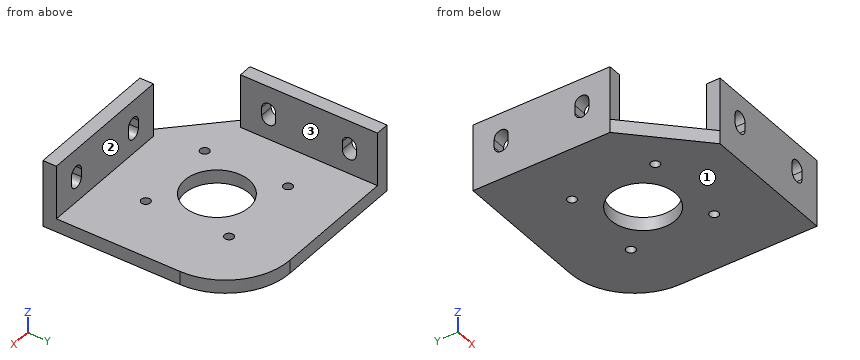
```python
from build123d import *

# Parameters (mm, degrees)
PAD_DEPTH       = 5
SKETCH002_R     = 1.68
SKETCH002_R_2   = 12
POCKET_DEPTH    = 5
FILLET_R        = 24
SKETCH_W        = 5
SKETCH_H        = 51
SKETCH_W_2      = 51
SKETCH_H_2      = 5
PAD001_DEPTH    = 20
POCKET001_DEPTH = 5
POCKET002_DEPTH = 5


with BuildPart() as part:
    # Sketch001 → Pad (new body)
    with BuildSketch(Plane.XY):
        Polygon((75, 0), (75, 75), (0, 75), (0, 24), (24, 0), align=None)
    extrude(amount=PAD_DEPTH)

    # Sketch002 → Pocket (cut)
    with BuildSketch(Plane(origin=(0, 0, 0), x_dir=(1, 0, 0), z_dir=(0, 0, -1))):
        with Locations((21, -22)):
            Circle(SKETCH002_R)
        with Locations((52, -22)):
            Circle(SKETCH002_R)
        with Locations((52, -53)):
            Circle(SKETCH002_R)
        with Locations((21, -53)):
            Circle(SKETCH002_R)
        with Locations((36.5, -37.5)):
            Circle(SKETCH002_R_2)
    extrude(amount=-POCKET_DEPTH, mode=Mode.SUBTRACT)

    # Fillet
    fillet_edges = [part.edges().sort_by_distance(p)[0] for p in [
        (75, 75, 2.5),
    ]]
    fillet(fillet_edges, radius=FILLET_R)

    # Sketch → Pad001 (new body)
    with BuildSketch(Plane.XY.offset(5)):
        with Locations((2.5, 49.5)):
            Rectangle(SKETCH_W, SKETCH_H)
        with Locations((49.5, 2.5)):
            Rectangle(SKETCH_W_2, SKETCH_H_2)
    extrude(amount=PAD001_DEPTH)

    # Sketch004 → Pocket001 (cut)
    with BuildSketch(Plane.YZ.offset(5)):
        with BuildLine():
            ThreePointArc((67.1, 16), (64.5, 18.6), (61.9, 16))
            Line((61.9, 16), (61.9, 13))
            ThreePointArc((61.9, 13), (64.5, 10.4), (67.1, 13))
            Line((67.1, 16), (67.1, 13))
        make_face()
        with BuildLine():
            ThreePointArc((37.1, 16), (34.5, 18.6), (31.9, 16))
            Line((31.9, 16), (31.9, 13))
            ThreePointArc((31.9, 13), (34.5, 10.4), (37.1, 13))
            Line((37.1, 16), (37.1, 13))
        make_face()
    extrude(amount=-POCKET001_DEPTH, mode=Mode.SUBTRACT)

    # Sketch003 → Pocket002 (cut)
    with BuildSketch(Plane(origin=(0, 5, 0), x_dir=(-1, 0, 0), z_dir=(0, 1, 0))):
        with BuildLine():
            ThreePointArc((-61.9, 16), (-64.5, 18.6), (-67.1, 16))
            Line((-67.1, 16), (-67.1, 13))
            ThreePointArc((-67.1, 13), (-64.5, 10.4), (-61.9, 13))
            Line((-61.9, 16), (-61.9, 13))
        make_face()
        with BuildLine():
            Line((-31.9, 16), (-31.9, 13))
            ThreePointArc((-37.1, 13), (-34.5, 10.4), (-31.9, 13))
            Line((-37.1, 16), (-37.1, 13))
            ThreePointArc((-31.9, 16), (-34.5, 18.6), (-37.1, 16))
        make_face()
    extrude(amount=-POCKET002_DEPTH, mode=Mode.SUBTRACT)


solid = part.part
```
Geometry check sheet. Reference: the model listing, model coordinates, mm. Face numbers are marked on the shaded views. A direction names the side the tool comes from. Give positions to 0.01 mm unless a question says otherwise; leave off trailing zeros. Loops run counter-clockwise (first coordinate to the right, second up) from the corner with the lowest first, then second, coordinate; pieces in that order, holes last. Notation, with made-up numbers: M 85,4 L 113,4 A7 cw 113,8 Z; hole C 46,-21 d2. An arc over 180 degrees is marked long. Answer as CSV lines item,"result".
Item 1: Cross-section at C-C on y = 64.5. Record the cut outline in (x, z), and give its area (3 significant figures).
Values:
outline,"M 0,0 L 70.84,0 L 70.84,5 L 5,5 L 5,10.4 L 0,10.4 Z; M 0,18.6 L 5,18.6 L 5,25 L 0,25 Z"
area,"413 mm²"
Item 2: Access from +Z, -Z, +X, -X, +Y, -Y to the whole of each face (thin tool, end or side, straight path). Record for the marked faces 1, 2 and 3.
Values:
face 1,"-Z, +X, -X, +Y, -Y"
face 2,"+Z, +X, -X, +Y"
face 3,"+Z, +X, +Y, -Y"
Item 3: Cross-section at A-A on z = 14.25. Record the cut outline in (x, y).
Values:
outline,"M 0,24 L 5,24 L 5,31.9 L 0,31.9 Z; M 0,37.1 L 5,37.1 L 5,61.9 L 0,61.9 Z; M 0,67.1 L 5,67.1 L 5,75 L 0,75 Z; M 24,0 L 31.9,0 L 31.9,5 L 24,5 Z; M 37.1,0 L 61.9,0 L 61.9,5 L 37.1,5 Z; M 67.1,0 L 75,0 L 75,5 L 67.1,5 Z"
Item 4: Cross-section at B-B on x = 52. Record the cut outline in (y, z), and give its area (3 significant figures).
Values:
outline,"M 0,0 L 20.32,0 L 20.32,5 L 5,5 L 5,25 L 0,25 Z; M 23.68,0 L 51.32,0 L 51.32,5 L 23.68,5 Z; M 54.68,0 L 74.98,0 L 74.98,5 L 54.68,5 Z"
area,"441 mm²"
Item 5: Material ranges on line 1 (Y direction, x = 36.5, z = 3.5); line 2 (X direction, y = 37.5, z = 3.75); line 3 (X direction, y = 54.5, z = 2), recorded low to high.
Values:
line 1,"y = 0 to 25.5, 49.5 to 75"
line 2,"x = 0 to 24.5, 48.5 to 75"
line 3,"x = 0 to 20.24, 21.76 to 51.24, 52.76 to 74.74"
Item 6: Depth check by flat-ended pin: P1, Ø1.5, axis at x = 9.5, y = 22, coming from the +Z side; P2, Ø2.5, axis at x = 3, z = 14.5, coming from the -Y side; P3, Ø5.5, axis at y = 1.5, z = 15.5, coming from the -X side. Enter the tip coordinate at first touch or a pass-through.
Values:
P1,"stops at z = 5"
P2,"stops at y = 24"
P3,"stops at x = 24"
